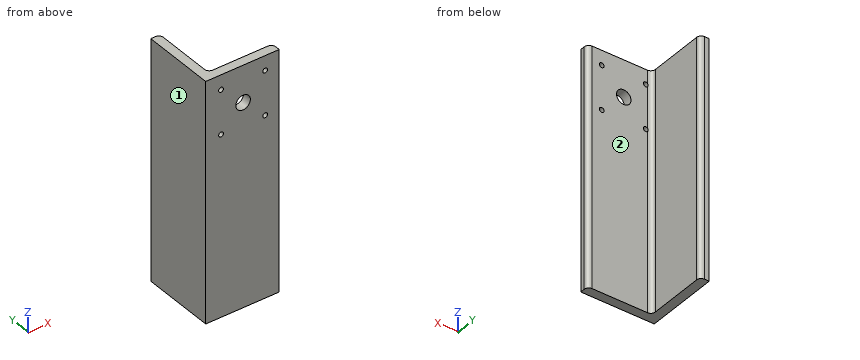
Autodesk Inventor part; units mm, degrees
ref_plane "YZ Plane" through (0, 0, 0) normal (1, 0, 0) x (0, 1, 0)
ref_plane "XZ Plane" through (0, 0, 0) normal (0, 1, 0) x (-1, 0, 0)
ref_plane "XY Plane" through (0, 0, 0) normal (0, 0, 1) x (1, 0, 0)
sketch "Sketch1" plane through (0, 0, 0) normal (0, 0, 1) x (1, 0, 0)
  line L0 (0, 0) -> (0, 50.8)
  line L1 (0, 0) -> (50.8, 0)
  line L2 (0, 50.8) -> (6.35, 50.8)
  line L3 (6.35, 50.8) -> (6.35, 0)
  line L4 (6.35, 0) -> (0, 0)
  line L5 (0, 0) -> (0, 50.8)
  line L6 (0, 0) -> (50.8, 0)
  line L7 (50.8, 0) -> (50.8, 6.35)
  line L8 (50.8, 6.35) -> (0, 6.35)
  line L9 (0, 6.35) -> (0, 0)
  dimension "d0" = 50.8
  dimension "d1" = 50.8
  dimension "d2" = 6.35
  dimension "d3" = 6.35
extrude "Extrusion1" add sketch "Sketch1" along normal blind 101.6
fillet "Fillet1" radius 3.175 1 edges at (6.35, 50.8, 50.8)
fillet "Fillet2" radius 3.175 1 edges at (50.8, 6.35, 50.8)
fillet "Fillet3" radius 3.175 1 edges at (6.35, 6.35, 50.8)
sketch "Sketch2" plane through (47.625, 6.35, 101.6) normal (0, 1, 0) x (1, 0, 0)
  circle A0 centre (-21.7932, 25.4) radius 5.0038
  line L0 (-47.625, 50.8) -> (-47.625, 101.6)
  line L1 (-47.625, 101.6) -> (-73.025, 101.6)
  line L2 (-73.025, 101.6) -> (-73.025, 0)
  line L3 (-73.025, 0) -> (3.6068, 0)
  line L4 (3.6068, 0) -> (3.6068, 50.8)
  line L5 (3.6068, 50.8) -> (-45.308, 50.8)
  line L6 (-45.308, 101.6) -> (-45.308, 50.8)
  line L7 (-45.4152, 101.6) -> (-45.308, 101.6)
  line L8 (-45.4152, 50.8) -> (-45.4152, 101.6)
  line L9 (-45.4152, 50.8) -> (-47.5178, 50.8)
  line L10 (-47.5178, 50.8) -> (-47.625, 50.8)
  circle A1 centre (-6.5659, 40.6273) radius 1.651
  circle A2 centre (-6.5659, 10.1727) radius 1.651
  circle A3 centre (-37.0205, 10.1727) radius 1.651
  circle A4 centre (-37.0205, 40.6273) radius 1.651
  line L11 (-38.1, 0) -> (-38.1, 101.6)
  line L12 (0, 0) -> (-38.1, 0)
  line L13 (0, 101.6) -> (0, 0)
  line L14 (0, 101.6) -> (-38.1, 101.6)
extrude "Extrusion2" cut sketch "Sketch2" along normal mid plane 25.4 contours A0 | L11 A3 | A3 L11 | L11 A4 | A4 L11 | A1 | A2
sketch "Sketch3" plane through (0, 0, 0) normal (0, 0, -1) x (-1, 0, 0)
  arc A0 (-47.625, 6.35) -> (-50.8, 3.175) centre (-47.625, 3.175) ccw
  line L0 (-50.8, 0) -> (-50.8, 3.175)
  line L1 (0, 0) -> (-50.8, 0)
  line L2 (0, 50.8) -> (0, 0)
  line L3 (-3.175, 50.8) -> (0, 50.8)
  arc A1 (-3.175, 50.8) -> (-6.35, 47.625) centre (-3.175, 47.625) ccw
  line L4 (-6.35, 9.525) -> (-6.35, 47.625)
  arc A2 (-9.525, 6.35) -> (-6.35, 9.525) centre (-9.525, 9.525) ccw
  line L5 (-47.625, 6.35) -> (-9.525, 6.35)
extrude "Extrusion3" add sketch "Sketch3" along normal blind 63.5
properties part number "L beam concept"
Can you work these out from the model? Positions are in its coordinate system, mm. Face numbers are marked on the shaded views. A direction names the side the tool comes from. Round coordinates to 2 decimals unless told otherwise and drop trailing zeros. Loops run counter-clockwise (first coordinate to the right, second up) from the corner with the lowest first, then second, coordinate; pieces in that order, holes last. Notation, with made-up numbers: M 6.5,-3 L 50.5,-3 A17 cw 50.5,14 Z; hole C 14,25.5 d10. An arc over 180 degrees is marked long. Write item = value, one per line. Start each with the question number.
(1) Suppose I cut it at A-A on z = 76.2. Write out the boundary of the cut face in (x, y) (3 decimals), plus the area to 3 significant figures.
(2) I need wall thicknesses on line 1 along X through (y, z) = (2, 76); line 2 along X through (y, z) = (36.5, 56). Which ranges of each line are inside material? Lowest first, please.
(3) Suppose I cut it at C-C on x = 33. Write out the boundary of the cut face in (y, z), plus the area to 3 significant figures.
(4) Which directions (+Z, -Z, +X, -X, +Y, -Y) give clear straight access to the entire face, cutting with the end or side of a thin tool? Please do the marked faces 1 and 2.
(5) Suppose I cut it at B-B on z = -46. Write out the boundary of the cut face in (x, y) (3 decimals).
(6) I'm going to push flat-ended pins straight in: P1, Ø1, axis at y = 5.5, z = -8, coming from the -X side; P2, Ø4.5, axis at x = 10.6, z = 91.43, coming from the +Y side; P3, Ø5, axis at y = 40, z = 53, coming from the +X side; P4, Ø1, axis at x = 42, z = 29, coming from the +Y side. Where does each tip first touch, or does it pass through?
Answer block:
q1.outline = M 0,0 L 20.828,0 L 20.828,6.35 L 9.525,6.35 A3.175 cw 6.35,9.525 L 6.35,47.625 A3.175 ccw 3.175,50.8 L 0,50.8 Z; M 30.836,0 L 50.8,0 L 50.8,3.175 A3.175 ccw 47.625,6.35 L 30.836,6.35 Z
q1.area = 539 mm²
q2.line_1 = 0 to 20.83, 30.83 to 50.8
q2.line_2 = 0 to 6.35
q3.outline = M 0,-63.5 L 6.35,-63.5 L 6.35,101.6 L 0,101.6 Z
q3.area = 1,050 mm²
q4.face_1 = +Z, -Z, -X, +Y, -Y
q4.face_2 = +Z, -Z, +X, +Y
q5.outline = M 0,0 L 50.8,0 L 50.8,3.175 A3.175 ccw 47.625,6.35 L 9.525,6.35 A3.175 cw 6.35,9.525 L 6.35,47.625 A3.175 ccw 3.175,50.8 L 0,50.8 Z
q6.P1 = 0
q6.P2 = 6.58
q6.P3 = 6.35
q6.P4 = 6.35
